from build123d import *

# Parameters (mm, degrees)
SKETCH_1_R      = 1.35
EXTRUDE_2_DEPTH = 3


with BuildPart() as part:
    # 草图1 → 凸台-拉伸2 (new body)
    with BuildSketch(Plane.XY):
        with BuildLine():
            Line((6.226098023, -5), (31.113248654, -5))
            ThreePointArc((31.113248654, -5), (36.113248654, -3.660254038), (39.773502692, 0))
            Line((39.773502692, 0), (51.622883551, 20.523729686))
            add(Edge.make_bspline(
                [(51.622883551, 20.523729686), (52.87217552, 21.925402984), (54.475191511, 21.032727874)],
                knots=[0, 0, 0, 1, 1, 1], degree=2))
            ThreePointArc((54.475191511, 21.032727874), (52.505149262, 29.672890493), (43.647343513, 29.942619722))
            add(Edge.make_bspline(
                [(40.471851368, 21.005877846), (44.982527223, 24.526926475), (43.647343513, 29.942619722)],
                knots=[0, 0, 0, 1, 1, 1], degree=2))
            Line((40.471851368, 21.005877846), (14.846921247, 4))
            Line((14.846921247, 4), (0, 4))
            ThreePointArc((0, 4), (-4, 0), (0, -4))
            Line((0, -4), (3.908343777, -4))
            add(Edge.make_bspline(
                [(3.908343777, -4), (4.94861431, -4.76744043), (6.226098023, -5)],
                knots=[0, 0, 0, 1, 1, 1], degree=2))
        make_face()
        Circle(SKETCH_1_R, mode=Mode.SUBTRACT)
        with Locations((34, 0)):
            Circle(SKETCH_1_R, mode=Mode.SUBTRACT)
    extrude(amount=EXTRUDE_2_DEPTH)


solid = part.part
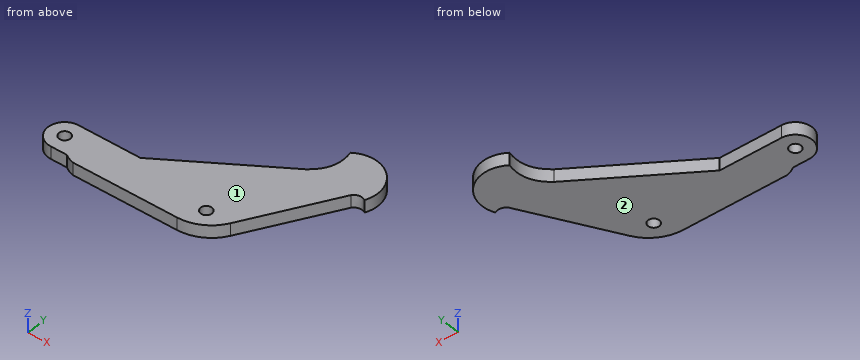
Geometry check sheet. Reference: the model listing, model coordinates, mm. Face numbers are marked on the shaded views. Give positions to 0.01 mm unless a question says otherwise; leave off trailing zeros. Write each loop counter-clockwise with the first axis right and the second up, starting at its lowest first coordinate (ties: lowest second). Pieces come first, ordered by that corner, then holes.
1) Release check for a two-part mould opening along Z. For the marked faces 1 and 2 record: released by +Z, released by -Z, zero draft, split by the parting line, or undercut.
Values follow:
face 1: released by +Z
face 2: released by -Z
2) Cross-section at C-C (x = 8). Record the boundary of the cut face in (y, z).
Values follow:
outline: (-5, 0) - (4, 0) - (4, 3) - (-5, 3) - close
3) Cross-section at D-D (x = 17). Record the boundary of the cut face in (y, z).
Values follow:
outline: (-5, 0) - (5.43, 0) - (5.43, 3) - (-5, 3) - close
4) Thickness scan on line 1 (Y direction, x = 0, z = 0.8); line 2 (X direction, y = 1, z = 1.75); line 3 (Y direction, x = 3.5, z = 2.1). Record the ranges inside material, lowest first.
Values follow:
line 1: y = -4 to -1.35, 1.35 to 4
line 2: x = -3.87 to -0.91, 0.91 to 33.09, 34.91 to 40.35
line 3: y = -4 to 4
5) Cross-section at A-A (x = 34). Record the boundary of the cut face in (y, z).
Values follow:
outline: (-4.57, 0) - (-1.35, 0) - (-1.35, 3) - (-4.57, 3) - close; (1.35, 0) - (16.71, 0) - (16.71, 3) - (1.35, 3) - close
6) Go/stop test with a flat-tipped pin: pin 1 Ø0.9 at (x, z) = (2, 2) entering from -Y. Record where the tip stops, or that it passes through.
Values follow:
pin 1: stops at y = -4
7) Cross-section at B-B (z = 1.6). Count the separate pieces of the cut face and the enclosed holes in it, plus the area to 3 significant figures.
Values follow:
separate pieces: 1
enclosed holes: 2
area: 796 mm2
